from build123d import *

# Parameters (mm, degrees)
SKETCH1_W           = 45
SKETCH1_H           = 13
MAIN_DEPTH          = 7
SKETCH4_W           = 45
SKETCH4_H           = 2.9
MAKERBEAMFIX_DEPTH  = 1
SKETCH5_R           = 1.5
MAKERBEAMHOLE_DEPTH = 9
SKETCH6_R           = 16
SKETCH6_R_2         = 10.1
MOTORFIX_DEPTH      = 3
SKETCH7_R           = 16
MOTORHOLE_DEPTH     = 10
SKETCH8_R           = 1.5
MOTORFIXHOLE_DEPTH  = 14
FILLET1_R           = 3


with BuildPart() as part:
    # Sketch1 → Main (new body)
    with BuildSketch(Plane.XY):
        Rectangle(SKETCH1_W, SKETCH1_H)
    extrude(amount=MAIN_DEPTH)

    # Sketch4 → MakerBeamFix (add)
    with BuildSketch(Plane.XY.offset(7)):
        with Locations((0, -1.5)):
            Rectangle(SKETCH4_W, SKETCH4_H)
    extrude(amount=MAKERBEAMFIX_DEPTH)

    # Sketch5 → MakerBeamHole (cut, through all)
    with BuildSketch(Plane.XY.offset(8)):
        with Locations((-19, -1.5)):
            Circle(SKETCH5_R)
        with Locations((19, -1.5)):
            Circle(SKETCH5_R)
    extrude(amount=-MAKERBEAMHOLE_DEPTH, mode=Mode.SUBTRACT)

    # Sketch6 → MotorFix (add)
    with BuildSketch(Plane(origin=(0, -6.5, 0), x_dir=(1, 0, 0), z_dir=(0, 1, 0))):
        with Locations((0, 11)):
            Circle(SKETCH6_R)
        with Locations((0, 11)):
            Circle(SKETCH6_R_2, mode=Mode.SUBTRACT)
    extrude(amount=MOTORFIX_DEPTH)

    # Sketch7 → MotorHole (cut)
    with BuildSketch(Plane(origin=(0, 6.5, 0), x_dir=(-1, 0, 0), z_dir=(0, -1, 0))):
        with Locations((0, 11)):
            Circle(SKETCH7_R)
    extrude(amount=MOTORHOLE_DEPTH, mode=Mode.SUBTRACT)

    # Sketch8 → MotorFixHole (cut, through all)
    with BuildSketch(Plane(origin=(0, 6.5, 0), x_dir=(1, 0, 0), z_dir=(0, 1, 0))):
        with Locations((9.192388155, 20.192388155)):
            Circle(SKETCH8_R)
        with Locations((-9.192388155, 20.192388155)):
            Circle(SKETCH8_R)
        with Locations((-9.192388155, 1.807611845)):
            Circle(SKETCH8_R)
        with Locations((9.192388155, 1.807611845)):
            Circle(SKETCH8_R)
    extrude(amount=-MOTORFIXHOLE_DEPTH, mode=Mode.SUBTRACT)

    # Fillet1
    fillet1_edges = [part.edges().sort_by_distance(p)[0] for p in [
        (-11.618950039, -5, 0),
        (11.618950039, -5, 0),
    ]]
    fillet(fillet1_edges, radius=FILLET1_R)


solid = part.part
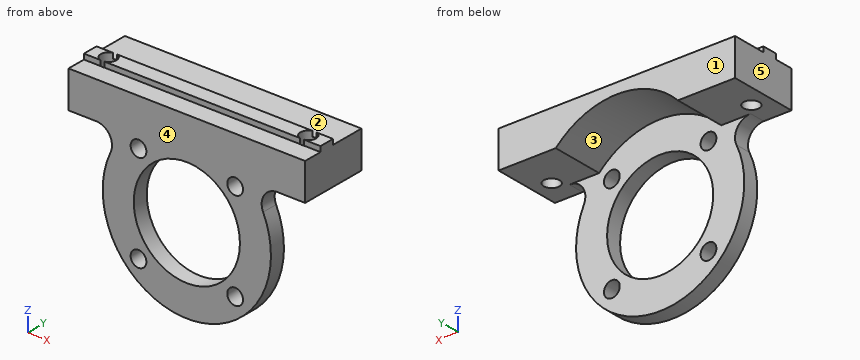
Could you check a few things on this model? Use its own coordinates, in mm. Face numbers are marked on the shaded views. A direction names the side the tool comes from. Coordinates: 2 decimals unless noted, no trailing zeros. Loops run counter-clockwise (first coordinate to the right, second up) from the corner with the lowest first, then second, coordinate; pieces in that order, holes last.
1. For the marked faces 1 and 2, which set-ups out of +Z, -Z, +X, -X, +Y, -Y let a thin tool reach every point of the face, with its end or its side?
2. Imagine slicing it at D-D (y = -5). Please give me the cut outline in (x, z).
3. We'd pull the mould along X, two halves only. Please class the marked faces 3, 4 and 5: released by +X, released by -X, zero draft, split by the parting line, or undercut.
4. Imagine slicing it at B-B (z = -11). Please give me the cut outline in (x, y), and give its area (3 significant figures).
5. I need wall thicknesses on L1, parallel to Z at x = 0, y = -4.7; L2, parallel to X at y = -2.25, z = 7; L3, parallel to Z at x = 15, y = -0.25. Which ranges of each line are inside material? Lowest first, please.
6. Imagine slicing it at A-A (y = -1.5). Please give me the cut outline in (x, z), and give its area (3 significant figures).
7. For P1, Ø0.5, axis at x = -3.5, z = 7.5, coming from the -Y side; P2, Ø0.8, axis at x = 21, z = 7.5, coming from the +Y side; P3, Ø3.5, axis at x = -19.5, y = -0.5, coming from the -Z side, each with a flat end and sliding along its axis, tell me the tip position at first contact or that it passes through.
8. Imagine slicing it at C-C (x = 0). Please give me the cut outline in (y, z), and give its area (3 significant figures).
Computed values:
1. face 1: +Z, -Z, +X, -X, +Y
1. face 2: +Z, +X, -X, +Y
2. outline: (-22.5, 0) - (-17.23, 0) arc R3 cw to (-14.51, -4.26) arc R16 ccw (long way) to (14.51, -4.26) arc R3 cw to (17.23, 0) - (22.5, 0) - (22.5, 7) - (-22.5, 7) - close; hole circle Ø3 at (-9.19, -20.19); hole circle Ø3 at (-9.19, -1.81); hole circle Ø20.2 at (0, -11); hole circle Ø3 at (9.19, -20.19); hole circle Ø3 at (9.19, -1.81)
3. face 3: undercut
3. face 4: zero draft
3. face 5: released by -X
4. outline: (-16, -6.5) - (-10.1, -6.5) - (-10.1, -3.5) - (-16, -3.5) - close; (10.1, -6.5) - (16, -6.5) - (16, -3.5) - (10.1, -3.5) - close
4. area: 35.4 mm2
5. L1: z = -27 to -21.1, -0.9 to 7
5. L2: x = -22.5 to -20.3, -17.7 to 17.7, 20.3 to 22.5
5. L3: z = 0 to 8
6. outline: (-22.5, 0) - (-20.5, 0) - (-20.5, 8) - (-22.5, 8) - close; (-17.5, 0) - (-11.62, 0) arc R16 cw to (11.62, 0) - (17.5, 0) - (17.5, 8) - (-17.5, 8) - close; (20.5, 0) - (22.5, 0) - (22.5, 8) - (20.5, 8) - close
6. area: 232 mm2
7. P1: stops at y = -2.95
7. P2: stops at y = -0.05
7. P3: stops at z = 0
8. outline: (-6.5, -27) - (-3.5, -27) - (-3.5, -21.1) - (-6.5, -21.1) - close; (-6.5, -0.9) - (-3.5, -0.9) - (-3.5, 5) - (6.5, 5) - (6.5, 7) - (-0.05, 7) - (-0.05, 8) - (-2.95, 8) - (-2.95, 7) - (-6.5, 7) - close
8. area: 64.3 mm2
